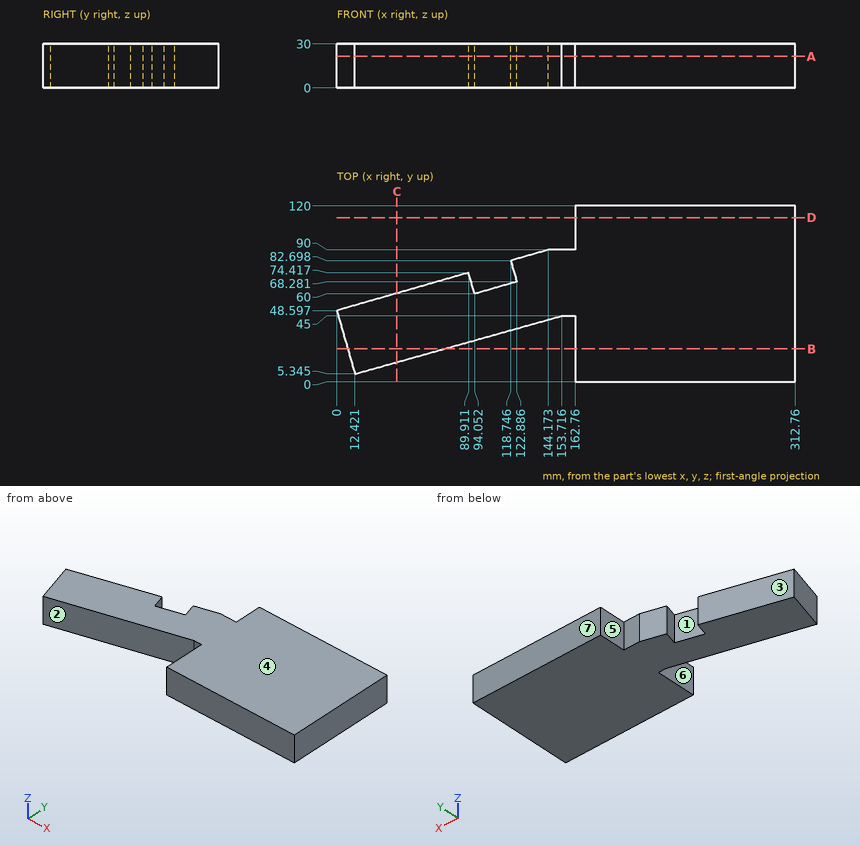
For this review, use the dimensioned drawing (mm, ordinates from the lowest corner) and the shaded views. A direction names the side the tool comes from. Round coordinates to 2 decimals unless told otherwise and drop trailing zeros. Order: outer loops, then holes, each group sorted by start corner. A loop starts at its lowest first (then second) coordinate and runs counter-clockwise, first axis right, second up.
1) Consider section A-A (z = 21.5). State the section outline as (x, y) points (1 decimal).
The answers:
outline: (0, 48.6) - (12.4, 5.3) - (153.7, 45) - (162.8, 45) - (162.8, 0) - (312.8, 0) - (312.8, 120) - (162.8, 120) - (162.8, 90) - (144.2, 90) - (118.7, 82.7) - (122.9, 68.3) - (94.1, 60) - (89.9, 74.4) - close
2) For L1, parallel to Y at x = 154, z = 28.5; L2, parallel to X at y = 93, z = 20.5; L3, parallel to Y at x = 100.5, z = 26.25 (1 decimal), list the stretches that pass through material, from the lowest coordinate up.
The answers:
L1: y = 45 to 90
L2: x = 162.76 to 312.76
L3: y = 30.1 to 61.9
3) Consider section B-B (y = 22.5). State the section outline as (x, z) points (1 decimal).
The answers:
outline: (7.5, 0) - (73.5, 0) - (73.5, 30) - (7.5, 30) - close; (162.8, 0) - (312.8, 0) - (312.8, 30) - (162.8, 30) - close
4) Consider section C-C (x = 41). State the section outline as (y, z) points (1 decimal).
The answers:
outline: (13.4, 0) - (60.4, 0) - (60.4, 30) - (13.4, 30) - close
5) Consider section D-D (y = 112). State the section outline as (x, z) points.
The answers:
outline: (162.76, 0) - (312.76, 0) - (312.76, 30) - (162.76, 30) - close
6) Clearance check with flat-ended pins moving along their axes: pin 1 Ø4 at (x, z) = (138.5, 7) entering from -Y; pin 2 Ø4 at (y, z) = (76.5, 17.5) entering from -X; pin 3 Ø1.5 at (x, z) = (46.5, 17.5) entering from -Y. State where each tip first meets the part, or that it passes through.
The answers:
pin 1: stops at y = 40.17
pin 2: stops at x = 119.95
pin 3: stops at y = 14.7
7) Draft analysis for pull direction X (two halves, no side actions). For the marked faces 1, 2, 3 and 4, state which applies: released by +X, released by -X, zero draft, split by the parting line, or undercut.
The answers:
face 1: undercut
face 2: undercut
face 3: released by -X
face 4: zero draft
8) Machinability: for the marked faces 5, 6 and 7, which of the approach directions +Z, -Z, +X, -X, +Y, -Y give a long, thin tool a straight path to every point of the face, cutting with its end or side? Answer none if there is none.
The answers:
face 5: +Z, -Z, -X, +Y
face 6: +Z, -Z, -Y
face 7: +Z, -Z, +X, -X, +Y
